Job drawing, mm, ordinate dimensions from the low corner. One solid piece. Give positions to 0.01 mm unless a question says otherwise; leave off trailing zeros. Loops run counter-clockwise (first coordinate to the right, second up) from the corner with the lowest first, then second, coordinate; pieces in that order, holes last.
Item 1: Probe probe 1 along Y at (x, z) = (27, 365.5); probe 2 along Z at (x, y) = (22.5, 1033.5). List the from-to ranges inside material, lowest first.
Item 2: Saw through at A-A on z = 2340. Give the cut face in (x, y).
Item 3: Saw through at C-C on y = 492. Give the cut face in (x, z).
Item 4: Saw through at B-B on x = 24. Give the cut face in (y, z).
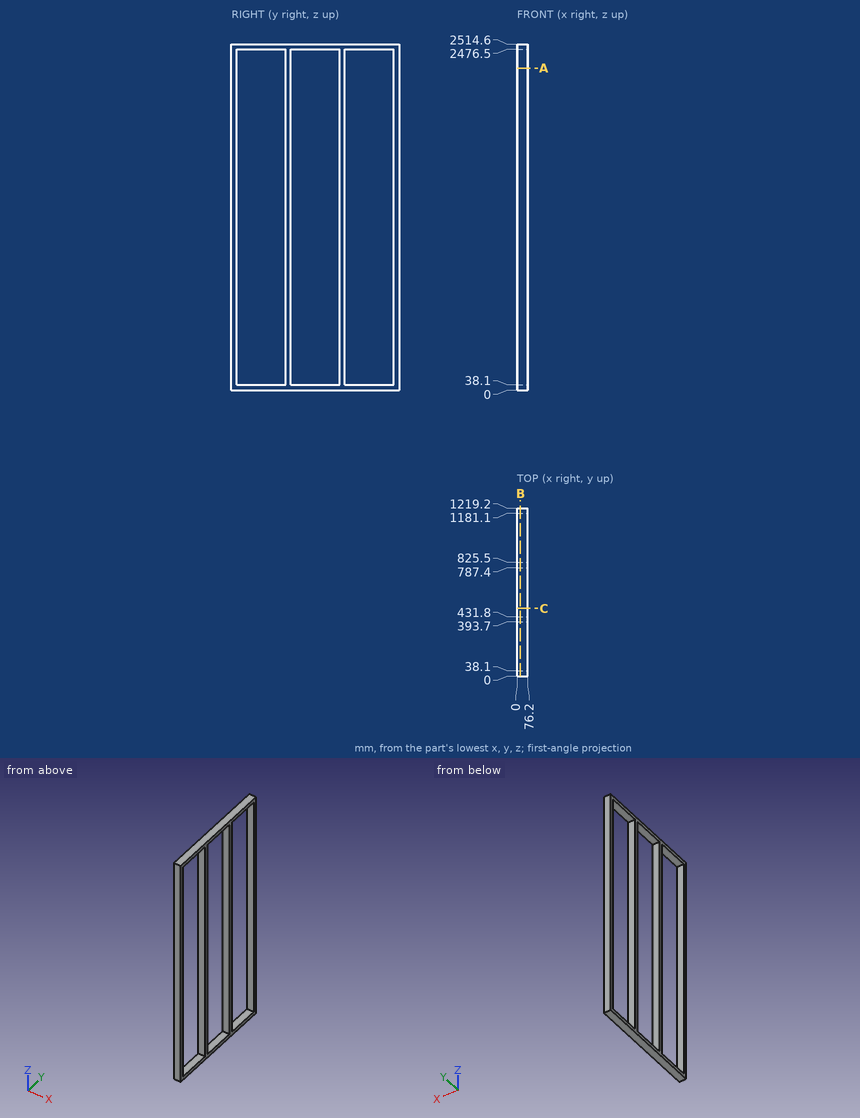
Results below:
1. probe 1: y = 0 to 38.1, 393.7 to 431.8, 787.4 to 825.5, 1181.1 to 1219.2
1. probe 2: z = 0 to 38.1, 2476.5 to 2514.6
2. outline: (0, 0) - (76.2, 0) - (76.2, 38.1) - (0, 38.1) - close; (0, 393.7) - (76.2, 393.7) - (76.2, 431.8) - (0, 431.8) - close; (0, 787.4) - (76.2, 787.4) - (76.2, 825.5) - (0, 825.5) - close; (0, 1181.1) - (76.2, 1181.1) - (76.2, 1219.2) - (0, 1219.2) - close
3. outline: (0, 0) - (76.2, 0) - (76.2, 38.1) - (0, 38.1) - close; (0, 2476.5) - (76.2, 2476.5) - (76.2, 2514.6) - (0, 2514.6) - close
4. outline: (0, 0) - (1219.2, 0) - (1219.2, 2514.6) - (0, 2514.6) - close; hole (38.1, 38.1) - (393.7, 38.1) - (393.7, 2476.5) - (38.1, 2476.5) - close; hole (431.8, 38.1) - (787.4, 38.1) - (787.4, 2476.5) - (431.8, 2476.5) - close; hole (825.5, 38.1) - (1181.1, 38.1) - (1181.1, 2476.5) - (825.5, 2476.5) - close
